Autodesk Fusion 360 part; units mm, degrees
sketch "Skizze1" plane through (0, 0, 0) normal (0, 0, 1) x (1, 0, 0)
  line L0 (0, 0) -> (53, 0)
  line L1 (53, 0) -> (53, 26)
  line L2 (53, 26) -> (0, 26)
  line L3 (0, 26) -> (0, 0)
  line L4 (1.6, 1.6) -> (51.4, 1.6)
  line L5 (51.4, 1.6) -> (51.4, 24.4)
  line L6 (51.4, 24.4) -> (1.6, 24.4)
  line L7 (1.6, 24.4) -> (1.6, 1.6)
  line L8 (3.4, 3.4) -> (49.6, 3.4)
  line L9 (49.6, 3.4) -> (49.6, 22.6)
  line L10 (49.6, 22.6) -> (3.4, 22.6)
  line L11 (3.4, 22.6) -> (3.4, 3.4)
  circle A0 centre (14.4, 7.6) radius 2
  line L12 (40.8, 20.25) -> (49.6, 20.25)
  line L13 (49.6, 20.25) -> (49.6, 5.75)
  line L14 (49.6, 5.75) -> (40.8, 5.75)
  line L15 (40.8, 5.75) -> (40.8, 20.25)
  line L16 (34.3, 22.6) -> (40.4, 22.6)
  line L17 (3.4, 8.5) -> (1.6, 8.5)
  line L18 (1.6, 8.5) -> (1.6, 17.5)
  line L19 (1.6, 17.5) -> (3.4, 17.5)
  line L20 (3.4, 17.5) -> (3.4, 8.5)
  line L21 (23.8, 8.2) -> (33.8, 8.2)
  line L22 (33.8, 8.2) -> (33.8, 18.2)
  line L23 (33.8, 18.2) -> (23.8, 18.2)
  line L24 (23.8, 18.2) -> (23.8, 8.2)
  line L25 (34.8, 1.6) -> (42.3, 1.6)
  line L26 (42.3, 1.6) -> (42.3, 8.8)
  line L27 (42.3, 8.8) -> (34.8, 8.8)
  line L28 (34.8, 8.8) -> (34.8, 1.6)
  dimension "d1" = 46.2
  dimension "d2" = 19.2
  dimension "d3" = 1.6
  dimension "d4" = 1.8
  dimension "d5" = 1.6
  dimension "d6" = 1.8
  dimension "d7" = 1.8
  dimension "d8" = 1.6
  dimension "d9" = 1.8
  dimension "d10" = 1.6
  dimension "d20" = 4
  dimension "d21" = 12.8
  dimension "d26" = 14.5
  dimension "d29" = 6
  dimension "d34" = 8.8
  dimension "d35" = 9
  dimension "d45" = 10
  dimension "d46" = 10
  dimension "d47" = 15.8
  dimension "d48" = 4.8
  dimension "d51" = 9.1
  dimension "d52" = 7.5
  dimension "d53" = 7.2
extrude "Extrusion1" add sketch "Skizze1" along normal blind 1.6 contours L0 L1 L2 L3 | L4 L7 L8 L11 L17 L28 | L4 L8 L25 L26 L28 | L7 L11 L17 L18 L19 L20 | L4 L5 L6 L7 L8 L9 L10 L11 L13 L16 L19 L26 | L8 L14 L15 L26 L27 L28 | L8 L9 L10 L11 L12 L15 L16 L20 L27 L28 | L8 L9 L14 L26 | L9 L12 L13 L14 L15 L26 L27 | L14 L15 L26 L27 | A0 | L21 L22 L23 L24
extrude "Extrusion2" add sketch "Skizze1" along normal blind 7 contours L0 L1 L2 L3
ref_plane "Arbeitsebene1" through (0, 13, 3.5) normal (-1, 0, 0) x (0, -1, 0)
sketch "Skizze2" plane through (0, 0, 0) normal (-1, 0, 0) x (0, -1, 0)
  line L0 (-20.5, 7) -> (-5.5, 7)
  line L1 (-5.5, 7) -> (-5.5, 0.8)
  line L2 (-5.5, 0.8) -> (-20.5, 0.8)
  line L3 (-20.5, 0.8) -> (-20.5, 7)
  line L4 (-26, 7) -> (0, 7)
  line L5 (-26, 0) -> (0, 0)
  dimension "d16" = 0.8
  dimension "d17" = 15
extrude "Extrusion3" cut sketch "Skizze2" against normal blind 1.6
extrude "Extrusion4" cut sketch "Skizze1" along normal blind 1.6 contours L4 L8 L25 L26 L28 | L8 L14 L15 L26 L27 L28 | L9 L12 L13 L14 L15 L26 L27 | L14 L15 L26 L27 | A0
extrude "Extrusion5" add sketch "Skizze1" along normal blind 2.6 contours L7 L11 L17 L18 L19 L20
ref_plane "Arbeitsebene2" through (1.6, 13, 1.7) normal (-1, 0, 0) x (0, 0, 1)
sketch "Skizze3" plane through (1.6, 0, 0) normal (-1, 0, 0) x (0, -1, 0)
  line L0 (-8.5, 2.6) -> (-17.5, 2.6)
  line L1 (-17, 2.1) -> (-9, 2.1)
  line L2 (-17.5, 2.6) -> (-8.5, 2.6)
  arc A0 (-9, 2.1) -> (-8.5, 2.6) centre (-9, 2.6) ccw
  arc A1 (-17.5, 2.6) -> (-17, 2.1) centre (-17, 2.6) ccw
  dimension "d39" = 0.5
  dimension "d41" = 0.5
  dimension "d42" = 0.5
extrude "Extrusion6" cut sketch "Skizze3" against normal blind 1.6
extrude "Extrusion7" add sketch "Skizze1" along normal blind 4 contours L21 L22 L23 L24
equation "d13 = 5.4 mm + 1.6 mm"
equation "d36 = 1.6 mm + 0.5 mm + 0.5 mm"
equation "d53 = 1.7 mm + 5.5 mm"
Design review of the part built by this model. Coordinates are the model's own, in mm. A direction names the side the tool comes from. Coordinates: 2 decimals unless noted, no trailing zeros. Write each loop counter-clockwise with the first axis right and the second up, starting at its lowest first coordinate (ties: lowest second). Pieces come first, ordered by that corner, then holes. Notation, with made-up numbers: (-9.5, -2) - (41.5, -2) arc R30 ccw to (41.5, 24) - close; hole circle Ø1 at (60.25, 54.25). An arc over 180 degrees is marked (long way). One line per item, written item: value.
1) Add section A-A (y = 12). State the section outline as (x, z) points.
Answer sheet:
outline: (0, 0) - (40.8, 0) - (40.8, 1.6) - (33.8, 1.6) - (33.8, 4) - (23.8, 4) - (23.8, 1.6) - (3.4, 1.6) - (3.4, 2.6) - (3.2, 2.6) - (3.2, 2.1) - (1.6, 2.1) - (1.6, 0.8) - (0, 0.8) - close; (49.6, 0) - (53, 0) - (53, 7) - (51.4, 7) - (51.4, 1.6) - (49.6, 1.6) - close
2) Mouldability with a two-part tool opening along Y and no side actions: class faces 4 (the face through (34.8, 5, 1)), 5 (the face through (28, 25, 7)) as +Y half, -Y half, draft (parallel to the pull), parting line (faces both ways), or undercut.
Answer sheet:
face 4: undercut
face 5: draft
3) Add section B-B (x = 14.4). State the section outline as (y, z) points, plus the area to 3 significant figures.
Answer sheet:
outline: (0, 0) - (5.6, 0) - (5.6, 1.6) - (1.6, 1.6) - (1.6, 7) - (0, 7) - close; (9.6, 0) - (26, 0) - (26, 7) - (24.4, 7) - (24.4, 1.6) - (9.6, 1.6) - close
area: 52.5 mm2
4) For faces 1 (the face through (45, 20.25, 1)), 2 (the face through (29, 8.2, 3)), 3 (the face through (1.6, 4, 4)), list the 3-axis set-ups (+Z, -Z, +X, -X, +Y, -Y) from which the entire face can be reached by the end or side of a thin tool; tool diameter is ignored.
Answer sheet:
face 1: +Z, -Z
face 2: +Z, -X
face 3: +Z
5) To check wall thickness, follow probe 1 along Y at (x, z) = (28.5, 2.25); probe 2 along Y at (x, z) = (14.4, 0.9); probe 3 along X at (y, z) = (2.75, 5). State the ranges of each line that lie inside material, in increasing order.
Answer sheet:
probe 1: y = 0 to 1.6, 8.2 to 18.2, 24.4 to 26
probe 2: y = 0 to 5.6, 9.6 to 26
probe 3: x = 0 to 1.6, 51.4 to 53
6) Add section C-C (y = 7.6). State the section outline as (x, z) points, plus the area to 3 significant figures.
Answer sheet:
outline: (0, 0) - (12.4, 0) - (12.4, 1.6) - (1.6, 1.6) - (1.6, 0.8) - (0, 0.8) - close; (16.4, 0) - (34.8, 0) - (34.8, 1.6) - (16.4, 1.6) - close; (49.6, 0) - (53, 0) - (53, 7) - (51.4, 7) - (51.4, 1.6) - (49.6, 1.6) - close
area: 62.1 mm2
7) Insertion check: pin 1 (2.5 mm diameter, centred on y = 14, z = 5.5, fed in from -X); pin 2 (4 mm diameter, centred on x = 12.5, y = 19.5, fed in from +Z); pin 3 (8 mm diameter, centred on x = 24, y = 15.5, fed in from +Z). Each pin has a flat end and moves straight along its axis. Give the tip position at first contact, or say it passes through.
Answer sheet:
pin 1: stops at x = 51.4
pin 2: stops at z = 1.6
pin 3: stops at z = 4
8) Add section D-D (x = 31.5). State the section outline as (y, z) points.
Answer sheet:
outline: (0, 0) - (26, 0) - (26, 7) - (24.4, 7) - (24.4, 1.6) - (18.2, 1.6) - (18.2, 4) - (8.2, 4) - (8.2, 1.6) - (1.6, 1.6) - (1.6, 7) - (0, 7) - close
